from build123d import *

# Parameters (mm, degrees)
SKETCH1_W                         = 76.2
SKETCH1_H                         = 50.8
BOSS_EXTRUDE1_DEPTH               = 6.35
F_1_4_20_TAPPED_HOLE1_D           = 5.1054
F_1_4_20_TAPPED_HOLE1_CSINK_D     = 7.62
F_1_4_20_TAPPED_HOLE1_CSINK_ANGLE = 90
F_3_8_16_TAPPED_HOLE1_D           = 7.9375


with BuildPart() as part:
    # Sketch1 → Boss-Extrude1 (new body)
    with BuildSketch(Plane(origin=(0, 0, 0), x_dir=(1, 0, 0), z_dir=(0, 1, 0))):
        with Locations((38.1, 25.4)):
            Rectangle(SKETCH1_W, SKETCH1_H)
    extrude(amount=BOSS_EXTRUDE1_DEPTH)

    # 1/4-20 Tapped Hole1 (through all)
    with Locations(Plane(origin=(0, 6.35, 0), x_dir=(1, 0, 0), z_dir=(0, 1, 0))):
        with Locations((17.905473556, 27.372280114), (57.470157442, 27.372280114)):
            CounterSinkHole(F_1_4_20_TAPPED_HOLE1_D / 2, F_1_4_20_TAPPED_HOLE1_CSINK_D / 2, counter_sink_angle=F_1_4_20_TAPPED_HOLE1_CSINK_ANGLE)

    # 3/8-16 Tapped Hole1 (through all)
    with Locations(Plane(origin=(0, 6.35, 0), x_dir=(1, 0, 0), z_dir=(0, 1, 0))):
        with Locations((34.599788687, 28.23429671)):
            Hole(F_3_8_16_TAPPED_HOLE1_D / 2)


solid = part.part
Could you check a few things on this model? Use its own coordinates, in mm. Coordinates: 2 decimals unless noted, no trailing zeros. Loops run counter-clockwise (first coordinate to the right, second up) from the corner with the lowest first, then second, coordinate; pieces in that order, holes last.
1. We'd pull the mould along Z, two halves only. Please class faces 1 (the face through (38, 3, 0)), 2 (the face through (37.52, 3.13, -30.92)), 3 (the face through (76.2, 3, -25)), 4 (the face through (55.035, 2.511, -28.139)): released by +Z, released by -Z, zero draft, split by the parting line, or undercut.
2. Imagine slicing it at A-A (x = 32). Please give me the cut outline in (y, z).
3. I need wall thicknesses on L1, parallel to X at y = 5.75, z = -26; L2, parallel to X at y = 3, z = -27; L3, parallel to X at y = 5, z = -31. Which ranges of each line are inside material? Lowest first, please.
4. Imagine slicing it at B-B (y = 4.25). Please give me the cut outline in (x, z), and give its area (3 significant figures).
5. For P1, Ø1, axis at x = 63, z = -31, coming from the -Y side; P2, Ø6.5, axis at x = 17.91, z = -27.37, coming from the +Y side, each with a flat end and sliding along its axis, tell me the tip position at first contact or that it passes through.
Computed values:
1. face 1: released by +Z
1. face 2: undercut
1. face 3: zero draft
1. face 4: undercut
2. outline: (0, -50.8) - (6.35, -50.8) - (6.35, -31.23) - (0, -31.23) - close; (0, -25.24) - (6.35, -25.24) - (6.35, 0) - (0, 0) - close
3. L1: x = 0 to 15, 20.81 to 31.32, 37.88 to 54.57, 60.37 to 76.2
3. L2: x = 0 to 15.38, 20.43 to 30.83, 38.37 to 54.94, 60 to 76.2
3. L3: x = 0 to 31.75, 37.45 to 76.2
4. outline: (0, -50.8) - (76.2, -50.8) - (76.2, 0) - (0, 0) - close; hole circle Ø5.11 at (17.91, -27.37); hole circle Ø7.94 at (34.6, -28.23); hole circle Ø5.11 at (57.47, -27.37)
4. area: 3,780 mm2
5. P1: stops at y = 0
5. P2: stops at y = 5.8
